CAD build for the part. Positions are in the model's coordinates, mm. A direction names the side the tool comes from. Round coordinates to 2 decimals unless told otherwise and drop trailing zeros. Loops run counter-clockwise (first coordinate to the right, second up) from the corner with the lowest first, then second, coordinate; pieces in that order, holes last. Notation, with made-up numbers: (84, 55) - (118, 55) arc R19 ccw to (118, 90) - close; hole circle Ø9 at (61, 60.5). An arc over 180 degrees is marked (long way). Use one line per item in the form item = value.
from build123d import *

# Parameters (mm, degrees)
F3_R            = 5
F4_DEPTH        = 4
F5_DEPTH        = 8
F5_COPIES_COUNT = 13
F5_COPIES_ANGLE = 324


# Not quite as in the source:
# - a feature of the source that left no trace in its solid (it failed there, or was rolled back) is left out
# - a pattern or mirror of a feature is missing from the dataset's text; its kind, count and spacing are read off the source's solid


with BuildPart() as f4:
    # F3 (on Front) → F4 (new body)
    with BuildSketch(Plane.XZ):
        with BuildLine():
            ThreePointArc((-2, 12.3389626793), (-8.100925873, -9.5197163823), (12.5, 0))
            ThreePointArc((12.5, 0), (9.5197163823, 8.100925873), (2, 12.3389626793))
            Line((2, 12.3389626793), (1.1255583585, 9.9364540145))
            Line((1.1255583585, 9.9364540145), (-1.1255583585, 9.9364540145))
            Line((-1.1255583585, 9.9364540145), (-2, 12.3389626793))
        make_face()
        Circle(F3_R, mode=Mode.SUBTRACT)
        with BuildLine():
            Line((1.1255583585, 9.9364540145), (2, 12.3389626793))
            ThreePointArc((2, 12.3389626793), (0, 12.5), (-2, 12.3389626793))
            Line((-2, 12.3389626793), (-1.1255583585, 9.9364540145))
            Line((-1.1255583585, 9.9364540145), (1.1255583585, 9.9364540145))
        make_face()
    extrude(amount=F4_DEPTH)

    # F3 (on Front) → F5 (cut)
    with BuildSketch(Plane.XZ):
        with BuildLine():
            Line((1.1255583585, 9.9364540145), (2, 12.3389626793))
            ThreePointArc((2, 12.3389626793), (0, 12.5), (-2, 12.3389626793))
            Line((-2, 12.3389626793), (-1.1255583585, 9.9364540145))
            Line((-1.1255583585, 9.9364540145), (1.1255583585, 9.9364540145))
        make_face()
    f5 = extrude(amount=F5_DEPTH, mode=Mode.SUBTRACT)

    # F5_copies: F5 ×13 about axis
    f5_copies_axis = Axis((0, 0, 0), (0, 1, 0))
    for i in range(1, F5_COPIES_COUNT):
        add(f5.rotate(f5_copies_axis, i * F5_COPIES_ANGLE / (F5_COPIES_COUNT - 1)), mode=Mode.SUBTRACT)


solid = f4.part
1) Drill centre lines: probe 1 along X at (y, z) = (-2.95, -0.25); probe 2 along X at (y, z) = (-1.6, 4); probe 3 along Z at (x, y) = (3, -2.7). Where is each one in solid material? Low to high.
Report:
probe_1 = -9.94 to -4.99, 4.99 to 12.5
probe_2 = -9.11 to -3, 3 to 11.84
probe_3 = -9.47 to -4, 4 to 12.13
2) Two-plate mould, pull along X, no slides. Class faces 1 (the cylindrical face through (-9.51, -1.97, -8.11)), 2 (the flat face through (0, 0, 6)), 3 (the flat face through (4.939, -1.972, -10.124)): +X half, -X half, draft (parallel to the pull), parting line (faces both ways), or undercut.
Report:
face_1 = -X half
face_2 = draft
face_3 = undercut
3) Tool access for faces 4 (the cylindrical face through (-12.15, -1.97, 2.93)), 5 (the flat face through (11.23, -1.97, 0.2)), 6 (the flat face through (3.666, -1.972, 10.651)), 7 (the flat face through (-9.936, -2, 0)), 8 (the flat face through (-0.195, -1.972, -11.263)): list every direction of +Z, -Z, +X, -X, +Y, -Y with a clear straight run to the whole face (end or side of a thin tool).
Report:
face_4 = +Z, -X, +Y, -Y
face_5 = +X, +Y, -Y
face_6 = +Y, -Y
face_7 = -X, +Y, -Y
face_8 = -Z, +Y, -Y
4) Flat gauge pins, fed straight in: pin 1 (1 mm diameter, centred on x = -2.5, y = -0.5, fed in from +Z); pin 2 (1.5 mm diameter, centred on x = 4.5, y = -3, fed in from +Z); pin 3 (0.7 mm diameter, centred on y = -3, z = 0, fed in from -X); pin 4 (1.8 mm diameter, centred on x = 0, y = -2.5, fed in from +Z). Where does each tip first touch, or does it go through?
Report:
pin_1 = 12.34
pin_2 = 11.92
pin_3 = -9.94
pin_4 = 9.94
5) Slice it at A-A (z = -8.25). Write the cut outline in (x, y), plus the area to 3 significant figures.
Report:
outline = (-9.39, -4) - (-8.05, -4) - (-8.05, 0) - (-9.39, 0) - close; (-5.55, -4) - (6.43, -4) - (6.43, 0) - (-5.55, 0) - close
area = 53.3 mm^2
6) Slice it at B-B (z = 1.5). Write the cut outline in (x, y).
Report:
outline = (-10.97, -4) - (-4.77, -4) - (-4.77, 0) - (-10.97, 0) - close; (4.77, -4) - (9.82, -4) - (9.82, 0) - (4.77, 0) - close
